```python
from build123d import *

# Parameters (mm, degrees)
SKETCH1_R           = 7.5
BOSS_EXTRUDE2_DEPTH = 25
FILLET2_R           = 3


with BuildPart() as part:
    # Sketch1 → Boss-Extrude2 (new body)
    with BuildSketch(Plane.XY):
        with BuildLine():
            Line((22.075429532, 20.314413872), (69.716953021, -31.457057418))
            ThreePointArc((69.716953021, -31.457057418), (70.236883802, -57.955206367), (44, -61.703293088))
            ThreePointArc((44, -61.703293088), (0, -48.516465442), (-44, -61.703293088))
            ThreePointArc((-44, -61.703293088), (-70.236883802, -57.955206367), (-69.716953021, -31.457057418))
            Line((-69.716953021, -31.457057418), (-22.075429532, 20.314413872))
            ThreePointArc((-22.075429532, 20.314413872), (0, 30), (22.075429532, 20.314413872))
        make_face()
        with Locations((55, -45)):
            Circle(SKETCH1_R, mode=Mode.SUBTRACT)
        with Locations((-55, -45)):
            Circle(SKETCH1_R, mode=Mode.SUBTRACT)
    extrude(amount=BOSS_EXTRUDE2_DEPTH)

    # Fillet2
    fillet2_edges = [part.edges().sort_by_distance(p)[0] for p in [
        (-70.236883802, -57.955206367, 25),
        (0, -48.516465442, 25),
        (70.236883802, -57.955206367, 25),
        (45.896191277, -5.571321773, 25),
        (0, 30, 25),
        (45.896191277, -5.571321773, 0),
        (70.236883802, -57.955206367, 0),
        (0, -48.516465442, 0),
        (-70.236883802, -57.955206367, 0),
        (-45.896191277, -5.571321773, 0),
        (0, 30, 0),
        (-45.896191277, -5.571321773, 25),
    ]]
    fillet(fillet2_edges, radius=FILLET2_R)


solid = part.part
```
Read the model definition and answer for the solid it produces. Units are mm, in the model's axes. Coordinates: 2 decimals unless noted, no trailing zeros. Write each loop counter-clockwise with the first axis right and the second up, starting at its lowest first coordinate (ties: lowest second). Pieces come first, ordered by that corner, then holes. Notation, with made-up numbers: (85.5, -33.5) - (113.5, -33.5) arc R28 ccw to (113.5, 4.5) - close; hole circle Ø11 at (55.5, 77). An arc over 180 degrees is marked (long way). Answer as a JSON object with one key per item and string values. Group by question number.
1. Each of these flat-tipped pins is pushed along its axis until it touches: P1, Ø4, axis at x = -49, z = 3, coming from the +Y side; P2, Ø3, axis at y = -10, z = 17.5, coming from the +X side; P3, Ø1.5, axis at y = 11, z = 7, coming from the -X side. Where does it stop, or does it pass through?
2. Consider L1, parallel to X at y = -46, z = 1; L2, parallel to Z at x = 17, y = 21.5; L3, parallel to Y at x = -55, z = 14. Determine where each line is inside the solid, lowest interval first. Write a range as [from, to].
3. A cutting plane is placed at A-A (z = 8.75). Determine the outline of the cut face in (x, y).
4. The mould has two halves that part along X. Classify faces 1 (the flat face through (1, -27, 25)), 2 (the cylindrical face through (-56.63, -52.32, 12.32)), 3 (the cylindrical face through (-44.93, -5.79, 0.9)), 4 (the cylindrical face through (0, 30, 12)): +X half, -X half, draft (parallel to the pull), parting line (faces both ways), or undercut.
Worked out:
{
 "1": {"P1": "stops at y = -6.77", "P2": "stops at x = 51.35", "P3": "stops at x = -31.34"},
 "2": {"L1": "x = [-74.21, -62.43], [-47.57, 47.57], [62.43, 74.21]", "L2": "z = [0.03, 24.97]", "L3": "y = [-65, -52.5], [-37.5, -15.46]"},
 "3": {"outline": "(-69.72, -31.46) arc R20 ccw to (-44, -61.7) arc R80 cw to (44, -61.7) arc R20 ccw to (69.72, -31.46) - (22.08, 20.31) arc R30 ccw to (-22.08, 20.31) - close; hole circle Ø15 at (-55, -45); hole circle Ø15 at (55, -45)"},
 "4": {"face 1": "draft", "face 2": "undercut", "face 3": "-X half", "face 4": "parting line"}
}
